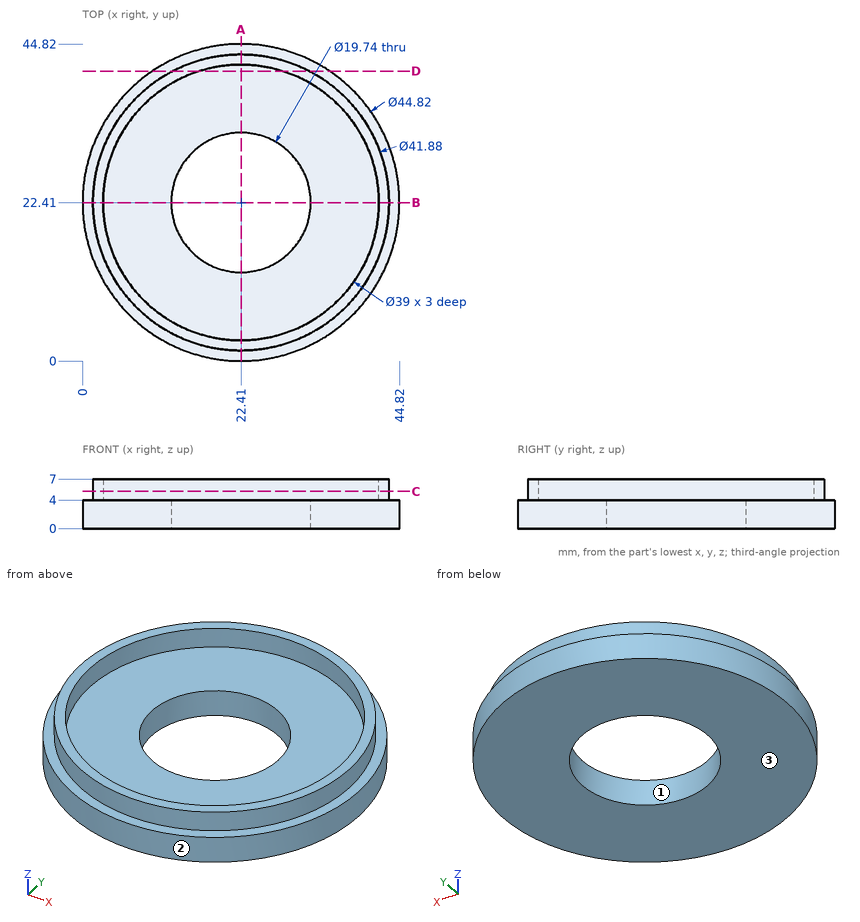
Could you check a few things on this drawing? It's one solid part, dimensions in mm from its lowest x, y, z. Coordinates: 2 decimals unless noted, no trailing zeros. Order: outer loops, then holes, each group sorted by start corner. A loop starts at its lowest first (then second) coordinate and runs counter-clockwise, first axis right, second up. Notation, with made-up numbers: M -32.5,54 L -1.5,54 A21 ccw -1.5,69 Z; hole C 54,-34.75 d5. An arc over 180 degrees is marked long. Use a Markdown table: item, result. Add a question column.
Q1. I want a section at C-C on z = 5.25. List the corners of the cut face in (x, y) for me.
Q2. I want a section at A-A on x = 22.41. List the corners of the cut face in (y, z) for me, then the cut area to 3 significant figures.
Q3. I'm going to push flat-ended pins straight in: pin 1 (6 mm diameter, centred on x = 20.5, y = 32.5, fed in from +Z); pin 2 (3 mm diameter, centred on y = 8.5, z = 0.5, fed in from -X). Where does each tip first touch, or does it pass through?
Q4. If I drill on L1, parallel to X at y = 22.41, z = 5.3; L2, parallel to Y at x = 22.41, z = 3.1, over which ranges is the centre line in solid material (lowest first)?
Q5. I want a section at D-D on y = 41. List the corners of the cut face in (x, z) for me.
Q6. We'd pull the mould along X, two halves only. Please class the marked faces 1, 2 and 3: pulls with the +X half, pulls with the -X half, needs draft (parallel to the pull), parting line crosses it, or undercut.
Checked values:
| question | item | result |
|---|---|---|
| 1 | outline | C 22.41,22.41 d41.88; hole C 22.41,22.41 d39 |
| 2 | outline | M 0,0 L 12.54,0 L 12.54,4 L 2.91,4 L 2.91,7 L 1.47,7 L 1.47,4 L 0,4 Z; M 32.28,0 L 44.82,0 L 44.82,4 L 43.35,4 L 43.35,7 L 41.91,7 L 41.91,4 L 32.28,4 Z |
| 2 | area | 109 mm² |
| 3 | pin 1 | z = 4 |
| 3 | pin 2 | x = 3.75 |
| 4 | L1 | 1.47 to 2.91, 41.91 to 43.35 |
| 4 | L2 | 0 to 12.54, 32.28 to 44.82 |
| 5 | outline | M 9.9,0 L 34.92,0 L 34.92,4 L 32.05,4 L 32.05,7 L 28.3,7 L 28.3,4 L 16.52,4 L 16.52,7 L 12.77,7 L 12.77,4 L 9.9,4 Z |
| 6 | face 1 | undercut |
| 6 | face 2 | parting line crosses it |
| 6 | face 3 | needs draft |
